Input: part model. Units: mm. Frame: model coordinates. Round coordinates to 2 decimals unless told otherwise and drop trailing zeros. Loops run counter-clockwise (first coordinate to the right, second up) from the corner with the lowest first, then second, coordinate; pieces in that order, holes last.
1) Section A-A, the plane y = 0. Return loops of the section in (x, z).
2) Ray query, line 1 along X through (y, z) = (5.5, 2); line 2 along Z through (x, y) = (-1.5, 3.75). Return the intervals inside material, ascending.
3) Section B-B, the plane x = -2.25. Return loops of the section in (y, z).
4) Section D-D, the plane y = -5.5. Return loops of the section in (x, z).
5) Section C-C, the plane z = 15.35. Return loops of the section in (x, y), and give its area (3 significant figures).
6) Draft query along Z for faces 1 (the face through (-2, 4, -18)), 2 (the face through (-2.46, 1.44, 10.77)), 3 (the face through (2, -15, -1)), 4 (the face through (2, 0, -40)). Return one class per face: pulls with the +Z half, pulls with the -Z half, needs draft (parallel to the pull), parting line crosses it, or undercut.
from build123d import *

# Parameters (mm, degrees)
SKETCH1_W           = 30
SKETCH1_H           = 80
SKETCH1_R           = 4.8
BOSS_EXTRUDE1_DEPTH = 5
SKETCH1_3_R         = 4.8
BOSS_EXTRUDE2_DEPTH = 5


with BuildPart() as part:
    # Sketch1 → Boss-Extrude1 (new body)
    # profile 1 of 3: a face of its own
    with BuildSketch(Plane.YZ):
        Rectangle(SKETCH1_W, SKETCH1_H)
        with Locations((0, -15.35)):
            Circle(SKETCH1_R, mode=Mode.SUBTRACT)
        with Locations((0, 15.35)):
            Circle(SKETCH1_R, mode=Mode.SUBTRACT)
    # profile 2 of 3: a face of its own
    with BuildSketch(Plane.YZ):
        with Locations((0, -15.35)):
            Circle(SKETCH1_R)
    # profile 3 of 3: a face of its own
    with BuildSketch(Plane.YZ):
        with Locations((0, 15.35)):
            Circle(SKETCH1_R)
    extrude(amount=BOSS_EXTRUDE1_DEPTH)

    # Sketch1_3 → Boss-Extrude2 (add)
    with BuildSketch(Plane.YZ):
        with Locations(Location((0, 15.35, 0), (0, 0, 270))):
            Circle(SKETCH1_3_R)
        with Locations(Location((0, -15.35, 0), (0, 0, 270))):
            Circle(SKETCH1_3_R)
    extrude(amount=-BOSS_EXTRUDE2_DEPTH)


solid = part.part
Final values:
1. outline: (-5, -20.15) - (0, -20.15) - (0, -40) - (5, -40) - (5, 40) - (0, 40) - (0, 20.15) - (-5, 20.15) - (-5, 10.55) - (0, 10.55) - (0, -10.55) - (-5, -10.55) - close
2. line 1: x = 0 to 5
2. line 2: z = -18.35 to -12.35, 12.35 to 18.35
3. outline: circle Ø9.6 at (0, -15.35); circle Ø9.6 at (0, 15.35)
4. outline: (0, -40) - (5, -40) - (5, 40) - (0, 40) - close
5. outline: (-5, -4.8) - (0, -4.8) - (0, -15) - (5, -15) - (5, 15) - (0, 15) - (0, 4.8) - (-5, 4.8) - close
5. area: 198 mm2
6. face 1: undercut
6. face 2: undercut
6. face 3: needs draft
6. face 4: pulls with the -Z half
